Source: CAD feature listing. Evaluate the final solid. Frame: model axes, mm. Face numbers are marked on the shaded views. A direction names the side the tool comes from. Give positions to 0.01 mm unless a question says otherwise; leave off trailing zeros. Order: outer loops, then holes, each group sorted by start corner. A loop starts at its lowest first (then second) coordinate and runs counter-clockwise, first axis right, second up.
from build123d import *

# Parameters (mm, degrees)
SKETCH1_R           = 30
SKETCH1_R_2         = 7
BOSS_EXTRUDE1_DEPTH = 10
FILLET1_R           = 10
FILLET2_R           = 20
CUT_EXTRUDE1_DEPTH  = 65


with BuildPart() as part:
    # Sketch1 → Boss-Extrude1 (new, symmetric)
    with BuildSketch(Plane(origin=(0, 0, 0), x_dir=(1, 0, 0), z_dir=(0, 1, 0))):
        with BuildLine():
            Line((128.063755469, 9.084385863), (27.935473676, 25.760615491))
            ThreePointArc((27.935473676, 25.760615491), (-38, 0), (27.935473676, -25.760615491))
            Line((27.935473676, -25.760615491), (128.063755469, -9.084385863))
            ThreePointArc((128.063755469, -9.084385863), (155, 0), (128.063755469, 9.084385863))
        make_face()
        with Locations(Location((0, 0, 0), (0, 0, 270))):
            Circle(SKETCH1_R, mode=Mode.SUBTRACT)
        with Locations(Location((140, 0, 0), (0, 0, 270))):
            Circle(SKETCH1_R_2, mode=Mode.SUBTRACT)
    extrude(amount=BOSS_EXTRUDE1_DEPTH, both=True)

    # Fillet1
    fillet1_edges = [part.edges().sort_by_distance(p)[0] for p in [
        (128.063755469, 0, 9.084385863),
        (128.063755469, 0, -9.084385863),
    ]]
    fillet(fillet1_edges, radius=FILLET1_R)

    # Fillet2
    fillet2_edges = [part.edges().sort_by_distance(p)[0] for p in [
        (27.935473676, 0, 25.760615491),
        (27.935473676, 0, -25.760615491),
    ]]
    fillet(fillet2_edges, radius=FILLET2_R)

    # Sketch2 → Cut-Extrude1 (cut)
    with BuildSketch(Plane(origin=(0, 10, 0), x_dir=(1, 0, 0), z_dir=(0, 1, 0))):
        with BuildLine():
            Line((42.150179221, 16.803642214), (107.507453416, 5.918476776))
            ThreePointArc((107.507453416, 5.918476776), (112.52173913, 0), (107.507453416, -5.918476776))
            Line((107.507453416, -5.918476776), (42.150179221, -16.803642214))
            ThreePointArc((42.150179221, -16.803642214), (37.596406424, -15.198680064), (36.523081969, -10.491162161))
            ThreePointArc((36.523081969, -10.491162161), (38, 0), (36.523081969, 10.491162161))
            ThreePointArc((36.523081969, 10.491162161), (37.596406424, 15.198680064), (42.150179221, 16.803642214))
        make_face()
    extrude(amount=-CUT_EXTRUDE1_DEPTH, mode=Mode.SUBTRACT)


solid = part.part
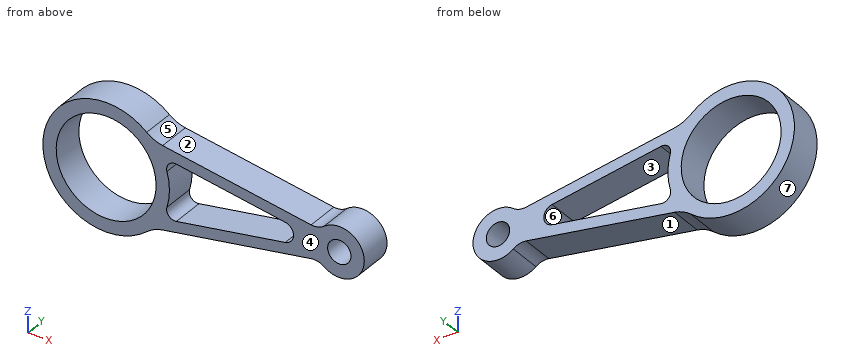
1) Section query A-A on x = 140. Output: boundary loops of the cut face in (y, z), and give its area (3 significant figures).
Checks:
outline: (-10, -15) - (10, -15) - (10, -7) - (-10, -7) - close; (-10, 7) - (10, 7) - (10, 15) - (-10, 15) - close
area: 320 mm2
2) First-contact query: pin 1 Ø1 at (x, y) = (121.5, -0.5) entering from -Z; pin 2 Ø2 at (y, z) = (-4.5, -15) entering from -X; pin 3 Ø11 at (x, z) = (140, 0) entering from +Y; pin 4 Ø8 at (x, y) = (129, -8) entering from +Z. Flat tips, straight axial feed; report the tip coordinate or a pass-through.
Checks:
pin 1: stops at z = -10.26
pin 2: stops at x = -35.33
pin 3: passes through
pin 4: stops at z = 13.27
3) Pull-direction query (Z, two-part tool) for the marked faces 5, 6 and 7; classes: +Z half, -Z half, draft (parallel to the pull), parting line (faces both ways), or undercut.
Checks:
face 5: +Z half
face 6: undercut
face 7: parting line
4) Section query D-D on x = 27. Output: boundary loops of the cut face in (y, z).
Checks:
outline: (-10, -27.29) - (10, -27.29) - (10, -13.08) - (-10, -13.08) - close; (-10, 13.08) - (10, 13.08) - (10, 27.29) - (-10, 27.29) - close
5) Section query B-B on z = 0. Output: boundary loops of the cut face in (x, y), and give its area (3 significant figures).
Checks:
outline: (-38, -10) - (-30, -10) - (-30, 10) - (-38, 10) - close; (30, -10) - (38, -10) - (38, 10) - (30, 10) - close; (112.52, -10) - (133, -10) - (133, 10) - (112.52, 10) - close; (147, -10) - (155, -10) - (155, 10) - (147, 10) - close
area: 890 mm2
6) Reachability of the marked faces 1, 2, 3 and 4 from +Z, -Z, +X, -X, +Y, -Y: full face, straight path, thin tool, end or side. Return the list, or none.
Checks:
face 1: -Z, +Y, -Y
face 2: +Z, +Y, -Y
face 3: +Y, -Y
face 4: +Z, -Z, +X, -X, -Y
7) Ray query, L1, parallel to Z at x = 59.5, y = 5.75; L2, parallel to X at y = 9, z = -2; L3, parallel to Z at x = -24, y = -1.25. Return the intervals inside material, ascending.
Checks:
L1: z = -20.5 to -13.91, 13.91 to 20.5
L2: x = -37.95 to -29.93, 29.93 to 37.95, 112.18 to 133.29, 146.71 to 154.87
L3: z = -29.46 to -18, 18 to 29.46
8) Section query C-C on y = 8. Output: boundary loops of the cut face in (x, z), and give its area (3 significant figures).
Checks:
outline: (24.38, -29.15) arc R20 cw to (33.92, -24.76) - (123.07, -9.92) arc R10 cw to (130.83, -11.87) arc R15 ccw (long way) to (130.83, 11.87) arc R10 cw to (123.07, 9.92) - (33.92, 24.76) arc R20 cw to (24.38, 29.15) arc R38 ccw (long way) to start; hole circle Ø60 at (0, 0); hole (36.52, -10.49) arc R5 ccw to (42.15, -16.8) - (107.51, -5.92) arc R6 ccw to (107.51, 5.92) - (42.15, 16.8) arc R5 ccw to (36.52, 10.49) arc R38 cw to start; hole circle Ø14 at (140, 0)
area: 3,680 mm2
